For this review, take the finished solid that the model builds, in its own axes (mm). A direction names the side the tool comes from. Coordinates: 2 decimals unless noted, no trailing zeros. Write each loop counter-clockwise with the first axis right and the second up, starting at its lowest first coordinate (ties: lowest second). Pieces come first, ordered by that corner, then holes.
```python
from build123d import *

# Parameters (mm, degrees)
SKETCH1_W           = 12.70451268
SKETCH1_H           = 8
SKETCH1_R           = 1
BOSS_EXTRUDE1_DEPTH = 8
CUT_EXTRUDE3_START  = -0.8
SKETCH4_R           = 3.25
CUT_EXTRUDE3_DEPTH  = 2.7
FILLET2_R           = 1
FILLET3_R           = 3


with BuildPart() as part:
    # Sketch1 → Boss-Extrude1 (new body)
    with BuildSketch(Plane.XY):
        with Locations((0.05225634, 0)):
            Rectangle(SKETCH1_W, SKETCH1_H)
        Circle(SKETCH1_R, mode=Mode.SUBTRACT)
        with Locations((5, 0)):
            Circle(SKETCH1_R, mode=Mode.SUBTRACT)
    extrude(amount=BOSS_EXTRUDE1_DEPTH)

    # Sketch4 → Cut-Extrude3 (cut)
    with BuildSketch(Plane.ZY.offset(6.3).offset(CUT_EXTRUDE3_START)):
        with Locations((4, 0)):
            Circle(SKETCH4_R)
    extrude(amount=-CUT_EXTRUDE3_DEPTH, mode=Mode.SUBTRACT)

    # Fillet2
    fillet2_edges = [part.edges().sort_by_distance(p)[0] for p in [
        (-6.3, -4, 4),
        (-6.3, 4, 4),
    ]]
    fillet(fillet2_edges, radius=FILLET2_R)

    # Fillet3
    fillet3_edges = [part.edges().sort_by_distance(p)[0] for p in [
        (6.40451268, 4, 4),
        (6.40451268, -4, 4),
    ]]
    fillet(fillet3_edges, radius=FILLET3_R)


solid = part.part
```
Q1. Add section A-A (y = 0). State the section outline as (x, z) points, then the cut area to 3 significant figures.
Ans:
outline: (-6.3, 0) - (-1, 0) - (-1, 8) - (-6.3, 8) - close; (1, 0) - (4, 0) - (4, 8) - (1, 8) - close; (6, 0) - (6.4, 0) - (6.4, 8) - (6, 8) - close; hole (-5.5, 0.75) - (-2.8, 0.75) - (-2.8, 7.25) - (-5.5, 7.25) - close
area: 52.1 mm2
Q2. For probe 1 along X at (y, z) = (-0.75, 5.75); probe 2 along Y at (x, z) = (-3.6, 4); probe 3 along X at (y, z) = (0.5, 0.5), list the stretches that pass through material, from the lowest coordinate up.
Ans:
probe 1: x = -6.3 to -5.5, -2.8 to -0.66, 0.66 to 4.34, 5.66 to 6.4
probe 2: y = -4 to -3.25, 3.25 to 4
probe 3: x = -6.3 to -0.87, 0.87 to 4.13, 5.87 to 6.4
Q3. Add section C-C (x = 0). State the section outline as (y, z) points, then the cut area to 3 significant figures.
Ans:
outline: (-4, 0) - (-1, 0) - (-1, 8) - (-4, 8) - close; (1, 0) - (4, 0) - (4, 8) - (1, 8) - close
area: 48.0 mm2
Q4. Add section D-D (z = 7.5). State the section outline as (x, y) points.
Ans:
outline: (-6.3, -3) arc R1 ccw to (-5.3, -4) - (3.4, -4) arc R3 ccw to (6.4, -1) - (6.4, 1) arc R3 ccw to (3.4, 4) - (-5.3, 4) arc R1 ccw to (-6.3, 3) - close; hole circle Ø2 at (0, 0); hole circle Ø2 at (5, 0)
Q5. Tool access review of faces 4 (the cylindrical face through (-4.17, 0.98, 7.1)), 5 (the flat face through (-1, -4, 4)): name each direction out of +Z, -Z, +X, -X, +Y, -Y from which nothing blocks a thin tool from reaching the whole face with its end or side.
Ans:
face 4: none
face 5: +Z, -Z, +X, -X, -Y
Q6. Add section B-B (z = 4). State the section outline as (x, y) points.
Ans:
outline: (-6.3, -3) arc R1 ccw to (-5.3, -4) - (3.4, -4) arc R3 ccw to (6.4, -1) - (6.4, 1) arc R3 ccw to (3.4, 4) - (-5.3, 4) arc R1 ccw to (-6.3, 3) - close; hole (-5.5, -3.25) - (-2.8, -3.25) - (-2.8, 3.25) - (-5.5, 3.25) - close; hole circle Ø2 at (0, 0); hole circle Ø2 at (5, 0)
Q7. Draft analysis for pull direction Z (two halves, no side actions). For faces 1 (the flat face through (-1.4, 0.1, 8)), 2 (the flat face through (-5.5, 0, 4)), 3 (the cylindrical face through (5.502, -3.145, 4.056)), state which applies: +Z half, -Z half, draft (parallel to the pull), parting line (faces both ways), or undercut.
Ans:
face 1: +Z half
face 2: undercut
face 3: draft
